from build123d import *

# Parameters (mm, degrees)
F1_DEPTH = 15
F2_W     = 40
F2_H     = 50
F3_DEPTH = 15
F5_R     = 5
F6_R     = 7.5
F7_DEPTH = 25
F8_R     = 3.1732892369
F9_DEPTH = 25
F10_R    = 0.5


with BuildPart() as f1:
    # F0 (on Top) → F1 (new body)
    with BuildSketch(Plane.XY):
        with BuildLine():
            ThreePointArc((-38.5634199679, -28.3495128886), (-37.0989538738, -31.8850467945), (-33.5634199679, -33.3495128886))
            Line((-33.5634199679, -33.3495128886), (21.4365800321, -33.3495128886))
            Line((21.4365800321, -33.3495128886), (21.4365800321, 66.6504871114))
            Line((21.4365800321, 66.6504871114), (-33.5634199679, 66.6504871114))
            ThreePointArc((-33.5634199679, 66.6504871114), (-37.0989538738, 65.1860210174), (-38.5634199679, 61.6504871114))
            Line((-38.5634199679, 61.6504871114), (-38.5634199679, -28.3495128886))
        make_face()
    extrude(amount=F1_DEPTH)


with BuildPart() as f3:
    # F2 (on face) → F3 (new body)
    with BuildSketch(Plane.YZ.offset(21.4365800321)):
        with Locations((16.6504871114, 40)):
            Rectangle(F2_W, F2_H)
    extrude(amount=-F3_DEPTH)

    # F4: union F1
    add(f1.part)

    # F5
    f5_edges = [f3.edges().sort_by_distance(p)[0] for p in [
        (6.43658, 16.650487, 15),
        (13.93658, -3.349513, 15),
        (13.93658, -3.349513, 65),
        (13.93658, 36.650487, 65),
        (13.93658, 36.650487, 15),
        (-6.06342, 66.650487, 15),
    ]]
    fillet(f5_edges, radius=F5_R)

    # F6 (on face) → F7 (cut)
    with BuildSketch(Plane(origin=(6.4365800321, 0, 0), x_dir=(0, -1, 0), z_dir=(-1, 0, 0))):
        with Locations((-16.6504871114, 50)):
            Circle(F6_R)
    extrude(amount=-F7_DEPTH, mode=Mode.SUBTRACT)

    # F8 (on face) → F9 (cut)
    with BuildSketch(Plane(origin=(0, 0, 0), x_dir=(1, 0, 0), z_dir=(0, 0, -1))):
        with Locations((-23.5634199679, -46.6504871114)):
            Circle(F8_R)
        with Locations((6.4365800321, -46.6504871114)):
            Circle(F8_R)
        with Locations((6.4365800321, 13.3495128886)):
            Circle(F8_R)
        with Locations((-23.5634199679, 13.3495128886)):
            Circle(F8_R)
    extrude(amount=-F9_DEPTH, mode=Mode.SUBTRACT)

    # F10
    f10_edges = [f3.edges().sort_by_distance(p)[0] for p in [
        (3.263291, -13.349513, 15),
        (-26.736709, -13.349513, 15),
        (-26.736709, 46.650487, 15),
        (3.263291, 46.650487, 15),
    ]]
    fillet(f10_edges, radius=F10_R)


solid = f3.part
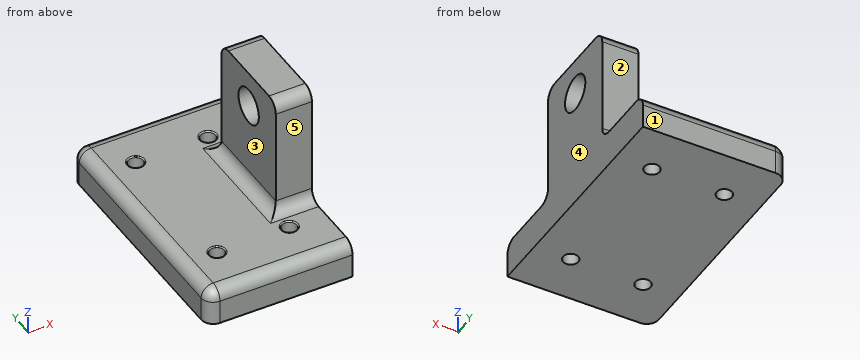
Model file for the job. Use its own axes, mm. Face numbers are marked on the shaded views. A direction names the side the tool comes from. Give positions to 0.01 mm unless a question says otherwise; leave off trailing zeros. Loops run counter-clockwise (first coordinate to the right, second up) from the corner with the lowest first, then second, coordinate; pieces in that order, holes last.
1) Saw through at B-B (x = 15). Write the cut outline in (y, z).
2) Saw through at D-D (y = 26.5). Write the cut outline in (x, z), plus the area to 3 significant figures.
3) Saw through at C-C (y = 14.5). Write the cut outline in (x, z).
4) Flat gauge pins, fed straight in: pin 1 Ø8 at (y, z) = (8, 42) entering from -X; pin 2 Ø5 at (x, y) = (-23.56, -13.35) entering from +Z; pin 3 Ø5 at (x, y) = (0, 31.5) entering from +Z; pin 4 Ø8 at (x, z) = (12, 13) entering from +Y. Where does each tip first touch, or does it go through?
5) Tool access for the marked faces 1, 2, 3, 4 and 5: list every direction of +Z, -Z, +X, -X, +Y, -Y with a clear straight run to the whole face (end or side of a thin tool).
6) Wall check: line 1 (X direction, y = 44, z = 13); line 2 (Y direction, x = -24, z = 4); line 3 (Z direction, x = 0, y = 17.5). Give the ranges that are in metal, low to high.
7) Saw through at A-A (z = 50). Write the cut outline in (x, y).
Answer block:
1. outline: (-33.35, 0) - (66.65, 0) - (66.65, 10) arc R5 ccw to (61.65, 15) - (41.65, 15) arc R5 cw to (36.65, 20) - (36.65, 60) arc R5 ccw to (31.65, 65) - (1.65, 65) arc R5 ccw to (-3.35, 60) - (-3.35, 20) arc R5 cw to (-8.35, 15) - (-28.35, 15) arc R5 ccw to (-33.35, 10) - close; hole circle Ø15 at (16.65, 50)
2. outline: (-38.56, 0) - (21.44, 0) - (21.44, 65) - (6.44, 65) - (6.44, 20) arc R5 cw to (1.44, 15) - (-33.56, 15) arc R5 ccw to (-38.56, 10) - close
2. area: 1,650 mm2
3. outline: (-38.56, 0) - (21.44, 0) - (21.44, 42.81) - (6.44, 42.81) - (6.44, 20) arc R5 cw to (1.44, 15) - (-33.56, 15) arc R5 ccw to (-38.56, 10) - close; (6.44, 57.19) - (21.44, 57.19) - (21.44, 65) - (6.44, 65) - close
4. pin 1: stops at x = 6.44
4. pin 2: passes through
4. pin 3: stops at z = 15.11
4. pin 4: stops at y = 66.65
5. face 1: +Z, -Z, +X, -X, +Y
5. face 2: +Z, +X, -X, +Y
5. face 3: +Z, -X, +Y, -Y
5. face 4: +Z, -Z, +X, +Y, -Y
5. face 5: +Z, +X, -X, -Y
6. line 1: x = -37.56 to -25.31, -21.82 to 4.69, 8.18 to 21.44
6. line 2: y = -33.35 to -16.49, -10.21 to 43.51, 49.79 to 66.65
6. line 3: z = 0 to 15
7. outline: (6.44, -3.35) - (21.44, -3.35) - (21.44, 9.15) - (6.44, 9.15) - close; (6.44, 24.15) - (21.44, 24.15) - (21.44, 36.65) - (6.44, 36.65) - close
